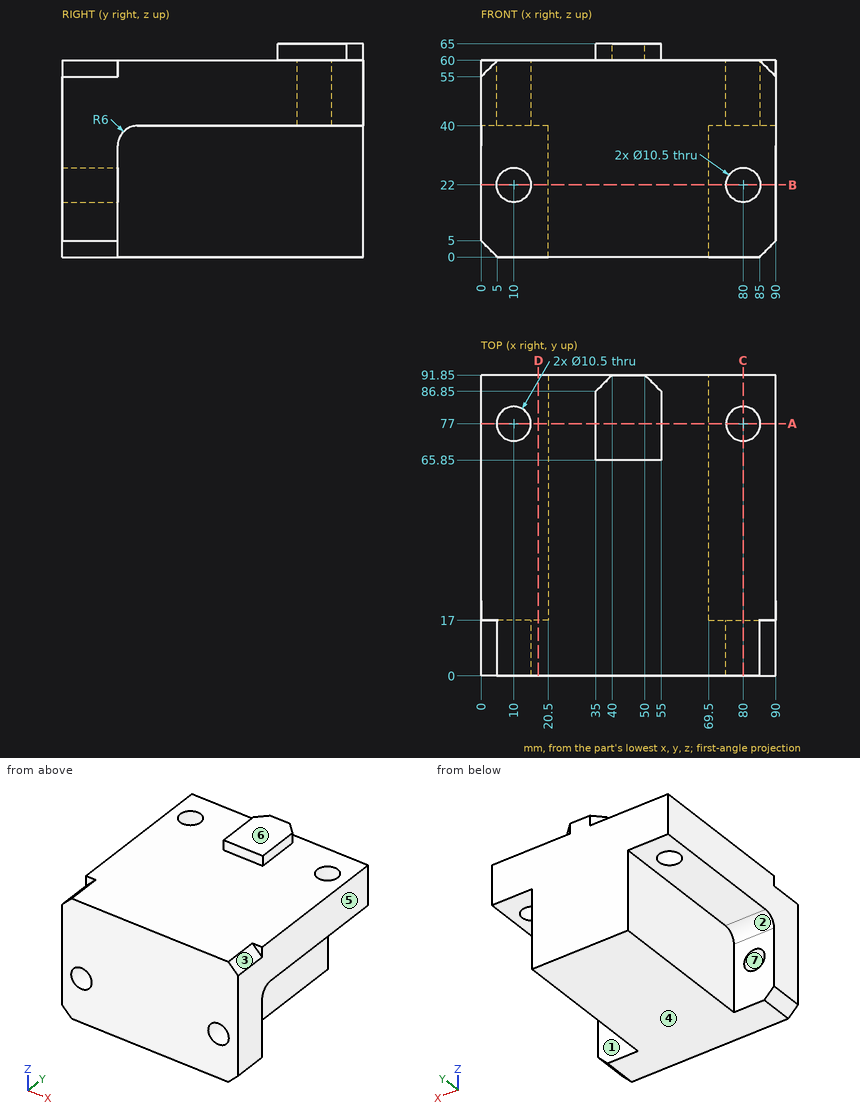
Check sheet for the drawn part. Datum: minimum x, y, z corner. Units: mm. A direction names the side the tool comes from. Give positions to 0.01 mm unless a question says otherwise; leave off trailing zeros. Loops run counter-clockwise (first coordinate to the right, second up) from the corner with the lowest first, then second, coordinate; pieces in that order, holes last. Notation, with made-up numbers: (85, -31.5) - (119, -31.5) arc R26 ccw to (119, 6.5) - close; hole circle Ø7 at (47.5, 16). An arc over 180 degrees is marked (long way). Write each question's results on one line, items separated by ' | '.
1) Sectioned sample at C-C on x = 80. Record the boundary of the cut face in (y, z).
Solution:
outline: (0, 0) - (17, 0) - (17, 16.75) - (0, 16.75) - close; (0, 27.25) - (17, 27.25) - (17, 34) arc R6 cw to (23, 40) - (71.75, 40) - (71.75, 60) - (0, 60) - close; (82.25, 40) - (91.85, 40) - (91.85, 60) - (82.25, 60) - close
2) Sectioned sample at A-A on y = 77. Record the boundary of the cut face in (x, z), plus the area to 3 significant figures.
Solution:
outline: (0, 40) - (4.75, 40) - (4.75, 60) - (0, 60) - close; (15.25, 40) - (20.5, 40) - (20.5, 0) - (69.5, 0) - (69.5, 40) - (74.75, 40) - (74.75, 60) - (55, 60) - (55, 65) - (35, 65) - (35, 60) - (15.25, 60) - close; (85.25, 40) - (90, 40) - (90, 60) - (85.25, 60) - close | area: 3,440 mm2
3) Tool access check on the marked faces 1, 2, 3 and 4. Record the directions out of +Z, -Z, +X, -X, +Y, -Y that give a thin tool (end or side, any length) a straight path to the whole face; none if there is none.
Solution:
face 1: -Z, +X, +Y | face 2: -Z, -X, +Y | face 3: +Z, +X, -Y | face 4: -Z, +X, -X, +Y, -Y
4) Mould release check, pull along Z, two halves, no side actions. Record for the marked faces 5, 6 and 7: pulls with the +Z half, pulls with the -Z half, needs draft (parallel to the pull), parting line crosses it, or undercut.
Solution:
face 5: needs draft | face 6: pulls with the +Z half | face 7: undercut
5) Depth check by flat-ended pin: P1, Ø10, axis at x = 70.5, y = 72, coming from the +Z side; P2, Ø5.5, axis at x = 41.5, z = 63.5, coming from the -Y side; P3, Ø13.5, axis at x = 10, y = 77, coming from the -Z side; P4, Ø2.5, axis at x = 3, z = 58.5, coming from the -Y side. Enter the tip coordinate at first touch or a pass-through.
Solution:
P1: z = 60 | P2: y = 65.85 | P3: z = 40 | P4: y = 0
6) Sectioned sample at D-D on x = 17.5. Record the boundary of the cut face in (y, z), plus the area to 3 significant figures.
Solution:
outline: (0, 0) - (17, 0) - (17, 34) arc R6 cw to (23, 40) - (91.85, 40) - (91.85, 60) - (0, 60) - close | area: 2,520 mm2
7) Sectioned sample at B-B on z = 22. Record the boundary of the cut face in (x, y), plus the area to 3 significant figures.
Solution:
outline: (0, 0) - (4.75, 0) - (4.75, 17) - (0, 17) - close; (15.25, 0) - (74.75, 0) - (74.75, 17) - (69.5, 17) - (69.5, 91.85) - (20.5, 91.85) - (20.5, 17) - (15.25, 17) - close; (85.25, 0) - (90, 0) - (90, 17) - (85.25, 17) - close | area: 4,840 mm2
8) Material ranges on L1, parallel to X at y = 77, z = 47.75; L2, parallel to Z at x = 80, y = 10.75; L3, parallel to Y at x = 10, z = 48, recorded low to high. Write a range as from..to.
Solution:
L1: 0..4.75, 15.25..74.75, 85.25..90 | L2: 0..16.75, 27.25..60 | L3: 0..71.75, 82.25..91.85
